For this review, take the finished solid that the model builds, in its own axes (mm). A direction names the side the tool comes from. Round coordinates to 2 decimals unless told otherwise and drop trailing zeros. Write each loop counter-clockwise with the first axis right and the second up, starting at its lowest first coordinate (ties: lowest second). Pieces come first, ordered by that corner, then holes. Notation, with made-up numbers: (39, 34) -> (77, 34) arc R35 cw to (77, 73) -> close; hole circle Ø6 at (78, 51.25). An arc over 180 degrees is marked (long way). Write item = value, one per line. Start each with the question number.
```python
from build123d import *

# Parameters (mm, degrees)
F0_W        = 9
F0_H        = 11
F2_DEPTH    = 70
F1_W        = 10
F1_H        = 1
F1_H_2      = 1.5
F3_DEPTH    = 40
F4_D        = 14.2875
F5_T1_DEPTH = 95.6598919876
F6_SIZE     = 5
F7_T1_DEPTH = 14.25
F7_T3_DEPTH = 33
F8_R        = 0.5


# Not quite as in the source:
# - a fillet or chamfer that OpenCascade refuses, or shapes differently, is made with other operations: its cross-section is extruded or revolved along the edge and cut away or added
# - a length typed as a fraction of an inch, garbled in the dataset ("3 / 203.2 mm" for 3/8 in), is restored


with BuildPart() as f2:
    # F0 (on Right) → F2 (new body)
    with BuildSketch(Plane.YZ):
        with Locations((-4.5, -5.5)):
            Rectangle(F0_W, F0_H)
        with Locations((4.5, -5.5)):
            Rectangle(F0_W, F0_H)
    extrude(amount=F2_DEPTH)

    # F1 (on Right) → F3 (join)
    with BuildSketch(Plane.YZ):
        with Locations((-5, -0.5)):
            Rectangle(F1_W, F1_H)
        with Locations((5, -0.5)):
            Rectangle(F1_W, F1_H)
        with Locations((5, 0.75)):
            Rectangle(F1_W, F1_H_2)
        with Locations((-5, 0.75)):
            Rectangle(F1_W, F1_H_2)
    extrude(amount=F3_DEPTH)

    # F4 (through all)
    with Locations(Plane(origin=(0, 0, 0), x_dir=(0, 1, 0), z_dir=(-1, 0, 0))):
        with Locations((0, 0)):
            Hole(F4_D / 2)

    # F5: chamfer of 15 x 8 on 1 edges, made by hand

    # F5_s2 → F5_t1 (cut)
    with BuildSketch(Plane.XZ.offset(-47.8299459938)):
        Polygon((55, -11), (70, -3), (70, -11), align=None)
    extrude(amount=F5_T1_DEPTH, mode=Mode.SUBTRACT)

    # F6
    f6_edges = [f2.edges().sort_by_distance(p)[0] for p in [
        (27.5, 9, -11),
        (27.5, -9, -11),
    ]]
    chamfer(f6_edges, length=F6_SIZE)

    # F7: fillet of radius 5 on 2 edges, made by hand

    # F7_s2 → F7_t1 (cut)
    with BuildSketch(Plane.XZ.offset(-7.125)):
        with BuildLine():
            ThreePointArc((53.75, -11), (54.9626781252, -10.8507125007), (56.1029411765, -10.4117647059))
            Line((56.1029411765, -10.4117647059), (55, -11))
            Line((55, -11), (53.75, -11))
        make_face()
    extrude(amount=F7_T1_DEPTH, mode=Mode.SUBTRACT)

    # F7_s4 → F7_t3 (cut)
    with BuildSketch(Plane.XZ.offset(-16.5)):
        with BuildLine():
            ThreePointArc((0, -6), (1.4644660941, -9.5355339059), (5, -11))
            Line((5, -11), (0, -11))
            Line((0, -11), (0, -6))
        make_face()
    extrude(amount=F7_T3_DEPTH, mode=Mode.SUBTRACT)

    # F8
    f8_edges = [f2.edges().sort_by_distance(p)[0] for p in [
        (20, -10, 1.5),
        (20, 10, 1.5),
        (20, -6.984495, 1.5),
        (20, 6.984495, 1.5),
    ]]
    fillet(f8_edges, radius=F8_R)


solid = f2.part
```
1. Consider section A-A, the plane z = -5.25. Give the boundary of the cut face in (x, y), then the cut area to 3 significant figures.
2. Clearance check with flat-ended pins moving along their axes: pin 1 Ø4 at (x, y) = (30, 1.5) entering from +Z; pin 2 Ø1 at (x, y) = (28, 7.5) entering from -Z; pin 3 Ø6 at (x, z) = (17, -8.5) entering from -Y. State where each tip first meets the part, or that it passes through.
3. Consider section C-C, the plane x = 38.5. Give the boundary of the cut face in (y, z).
4. Consider section D-D, the plane y = 0. Give the boundary of the cut face in (x, z), then the cut area to 3 significant figures.
5. Machinability: for faces 1 (the cylindrical face through (54.946, 0.064, -10.855)), 2 (the flat face through (55, 8, 0)), which of the approach directions +Z, -Z, +X, -X, +Y, -Y give a long, thin tool a straight path to every point of the face, cutting with its end or side? Answer none if there is none.
6. Consider section B-B, the plane y = -8.25. Give the boundary of the cut face in (x, z), then the cut area to 3 significant figures.
7. Wall thickness on L1, parallel to Z at x = 5, y = 3; L2, parallel to Y at x = 43, z = -5.25; L3, parallel to X at y = 7.5, z = 1: over which ranges is each line inside the solid? List them lowest first. Write a range as from..to.
Outcome:
q1.outline = (0, -9) -> (65.78, -9) -> (65.78, -4.84) -> (0, -4.84) -> close; (0, 4.84) -> (65.78, 4.84) -> (65.78, 9) -> (0, 9) -> close
q1.area = 547 mm2
q2.pin_1 = -6.23
q2.pin_2 = -8
q2.pin_3 = -9
q3.outline = (-10, -1) -> (-9, -1) -> (-9, -6) -> (-4, -11) -> (4, -11) -> (9, -6) -> (9, -1) -> (10, -1) -> (10, 1) arc R0.5 ccw to (9.5, 1.5) -> (7.58, 1.5) arc R0.5 ccw to (7.08, 0.93) arc R7.14 cw (long way) to (-7.08, 0.93) arc R0.5 ccw to (-7.58, 1.5) -> (-9.5, 1.5) arc R0.5 ccw to (-10, 1) -> close
q4.outline = (0.13, -7.14) arc R5 ccw to (5, -11) -> (53.75, -11) arc R5 ccw to (56.1, -10.41) -> (62.23, -7.14) -> close
q4.area = 221 mm2
q5.face_1 = -Z, +X, +Y, -Y
q5.face_2 = +Z, +X, +Y, -Y
q6.outline = (0, -6) arc R5 ccw to (0.06, -6.75) -> (62.97, -6.75) -> (70, -3) -> (70, 0) -> (40, 0) -> (40, 1.5) -> (0, 1.5) -> close
q6.area = 519 mm2
q7.L1 = -11..-6.48
q7.L2 = -9..-4.84, 4.84..9
q7.L3 = 0..40
